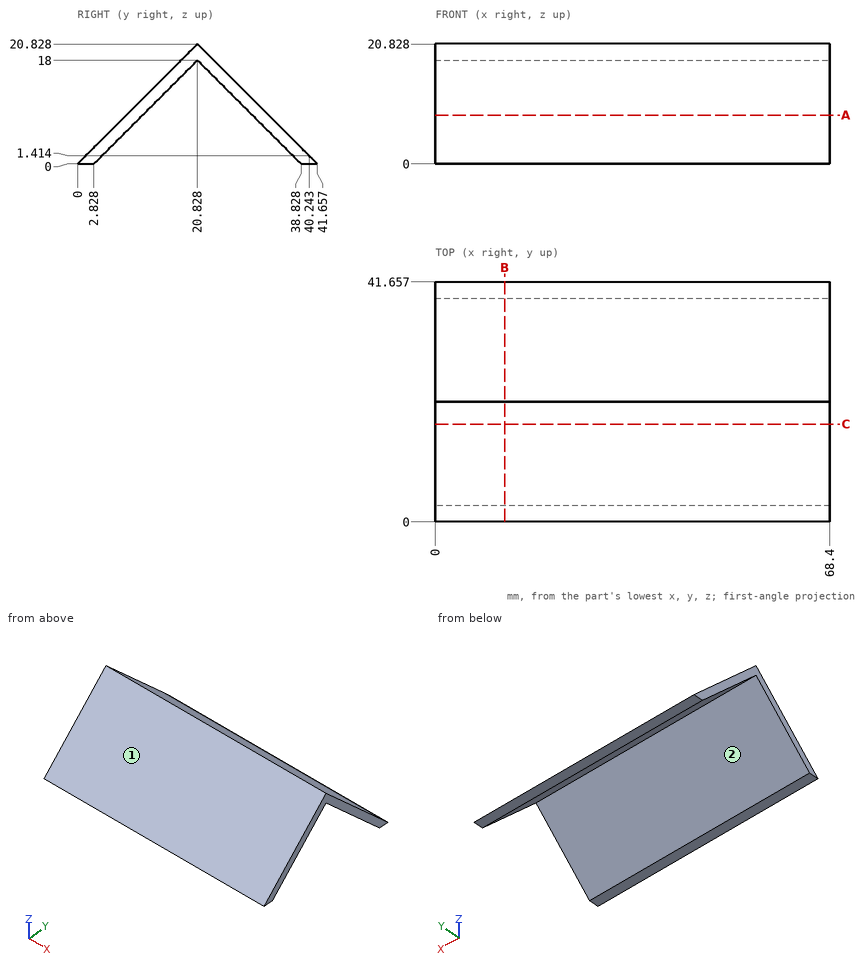
The drawing under review shows one solid part. Ordinate dimensions are in mm from its lowest x, y, z. Coordinates: 2 decimals unless noted, no trailing zeros. Write each loop counter-clockwise with the first axis right and the second up, starting at its lowest first coordinate (ties: lowest second). Pieces come first, ordered by that corner, then holes. Notation, with made-up numbers: (75.25, 41.25) -> (119.25, 41.25) arc R21 ccw to (119.25, 55.25) -> close; hole circle Ø6 at (-1, -14). An arc over 180 degrees is marked (long way). One line per item, written item: value. Start each with the question number.
Q1. Add section A-A, the plane z = 8.5. Give the boundary of the cut face in (x, y), then the cut area to 3 significant figures.
Q2. Add section B-B, the plane x = 12. Give the boundary of the cut face in (y, z) (1 decimal).
Q3. To check wall thickness, follow probe 1 along Y at (x, z) = (17, 7.5) (1 decimal); probe 2 along Y at (x, z) = (35.5, 6.5) (1 decimal); probe 3 along Z at (x, y) = (10, 25) (1 decimal). State the ranges of each line that lie inside material, in increasing order.
Q4. Add section C-C, the plane y = 17. Give the boundary of the cut face in (x, z).
Q5. Clearance check with flat-ended pins moving along their axes: P1, Ø1.5, axis at x = 12, z = 14.5, coming from the -Y side; P2, Ø1.5, axis at x = 11, z = 6, coming from the -Y side; P3, Ø10, axis at x = 26, y = 21.5, coming from the -Z side. State where each tip first meets the part, or that it passes through.
Q6. The part is to be moulded in two halves that separate along Y. For the marked faces 1 and 2, say which applies: +Y half, -Y half, draft (parallel to the pull), parting line (faces both ways), or undercut.
Response:
1. outline: (0, 8.5) -> (68.4, 8.5) -> (68.4, 11.33) -> (0, 11.33) -> close; (0, 30.33) -> (68.4, 30.33) -> (68.4, 33.16) -> (0, 33.16) -> close
1. area: 387 mm²
2. outline: (0, 0) -> (2.8, 0) -> (20.8, 18) -> (38.8, 0) -> (41.7, 0) -> (20.8, 20.8) -> close
3. probe 1: 7.5 to 10.3, 31.3 to 34.2
3. probe 2: 6.5 to 9.3, 32.3 to 35.2
3. probe 3: 13.8 to 16.7
4. outline: (0, 14.17) -> (68.4, 14.17) -> (68.4, 17) -> (0, 17) -> close
5. P1: y = 13.75
5. P2: y = 5.25
5. P3: z = 12.33
6. face 1: -Y half
6. face 2: undercut
